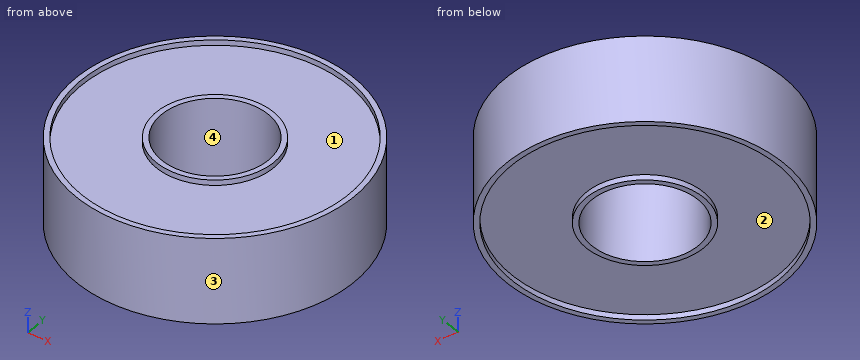
```python
from build123d import *

# Parameters (mm, degrees)
SKETCH1_R           = 13
SKETCH1_R_2         = 5
BOSS_EXTRUDE1_DEPTH = 8
SKETCH2_R           = 12.5
SKETCH2_R_2         = 5.5
CUT_EXTRUDE1_DEPTH  = 0.5


with BuildPart() as part:
    # Sketch1 → Boss-Extrude1 (new body)
    with BuildSketch(Plane.XY):
        Circle(SKETCH1_R)
        Circle(SKETCH1_R_2, mode=Mode.SUBTRACT)
    extrude(amount=BOSS_EXTRUDE1_DEPTH)

    # Sketch2 → Cut-Extrude1 (cut)
    with BuildSketch(Plane.XY.offset(8)):
        Circle(SKETCH2_R)
        Circle(SKETCH2_R_2, mode=Mode.SUBTRACT)
    cut_extrude1 = extrude(amount=-CUT_EXTRUDE1_DEPTH, mode=Mode.SUBTRACT)

    # Mirror1: Cut-Extrude1 across plane
    add(cut_extrude1.mirror(Plane(origin=(0, 0, 4), x_dir=(1, 0, 0), z_dir=(0, 0, -1))), mode=Mode.SUBTRACT)


solid = part.part
```
The listing builds one solid part. Answer for the finished solid, in the listing's coordinates (mm). Face numbers are marked on the shaded views. A direction names the side the tool comes from. Give positions to 0.01 mm unless a question says otherwise; leave off trailing zeros. Write each loop counter-clockwise with the first axis right and the second up, starting at its lowest first coordinate (ties: lowest second). Pieces come first, ordered by that corner, then holes. Notation, with made-up numbers: (-17.75, 4.5) -> (27.25, 4.5) arc R13 ccw to (27.25, 15.5) -> close; hole circle Ø11 at (-1, 61.5). An arc over 180 degrees is marked (long way). Write item = value, one per line. Start each with the question number.
1) The part is cut by section A-A, the plane y = 0. Determine the outline of the cut face in (x, z).
2) The part is cut by section C-C, the plane z = 5.25. Determine the outline of the cut face in (x, y).
3) Which of the six approach directions +Z, -Z, +X, -X, +Y, -Y give full straight-line access (tool end or side, diameter ignored) to the marked faces 1 and 2?
4) Each of these flat-tipped pins is pushed along its axis until it touches: pin 1 (1.5 mm diameter, centred on x = -7.5, z = 2, fed in from -Y); pin 2 (6 mm diameter, centred on x = 0, y = 0, fed in from -Z); pin 3 (3 mm diameter, centred on x = 6.5, z = 5.5, fed in from +Y). Where does it stop, or does it pass through?
5) The part is cut by section D-D, the plane y = 10.75. Determine the outline of the cut face in (x, z).
6) Straight lines are drawn through the part: line 1 along Y through (x, z) = (0, 0.25); line 2 along X through (y, z) = (-0.25, 3.75); line 3 along Y through (x, z) = (0, 4.5). For each, find the intervals that lie inside material, in ascending order.
7) Determine the mould class of the marked faces 3 and 4 for opening direction X: +X half, -X half, draft (parallel to the pull), parting line (faces both ways), or undercut.
Solutions:
q1.outline = (-13, 0) -> (-12.5, 0) -> (-12.5, 0.5) -> (-5.5, 0.5) -> (-5.5, 0) -> (-5, 0) -> (-5, 8) -> (-5.5, 8) -> (-5.5, 7.5) -> (-12.5, 7.5) -> (-12.5, 8) -> (-13, 8) -> close; (5, 0) -> (5.5, 0) -> (5.5, 0.5) -> (12.5, 0.5) -> (12.5, 0) -> (13, 0) -> (13, 8) -> (12.5, 8) -> (12.5, 7.5) -> (5.5, 7.5) -> (5.5, 8) -> (5, 8) -> close
q2.outline = circle Ø26 at (0, 0); hole circle Ø10 at (0, 0)
q3.face_1 = +Z
q3.face_2 = -Z
q4.pin_1 = -11.11
q4.pin_2 = through
q4.pin_3 = 12
q5.outline = (-7.31, 0) -> (-6.38, 0) -> (-6.38, 0.5) -> (6.38, 0.5) -> (6.38, 0) -> (7.31, 0) -> (7.31, 8) -> (6.38, 8) -> (6.38, 7.5) -> (-6.38, 7.5) -> (-6.38, 8) -> (-7.31, 8) -> close
q6.line_1 = -13 to -12.5, -5.5 to -5, 5 to 5.5, 12.5 to 13
q6.line_2 = -13 to -4.99, 4.99 to 13
q6.line_3 = -13 to -5, 5 to 13
q7.face_3 = parting line
q7.face_4 = undercut
